Check sheet for the modelled part. Datum: model origin and axes. Units: mm. A direction names the side the tool comes from. Round coordinates to 2 decimals unless told otherwise and drop trailing zeros. Write each loop counter-clockwise with the first axis right and the second up, starting at its lowest first coordinate (ties: lowest second). Pieces come first, ordered by that corner, then holes. Notation, with made-up numbers: M 82,34 L 116,34 A23 ccw 116,53 Z; hole C -29,-17.5 d9. An arc over 180 degrees is marked long. One line per item, written item: value.
from build123d import *

# Parameters (mm, degrees)
BOSS_EXTRUDE1_DEPTH     = 6.35
SKETCH3_R               = 2.286
CUT_EXTRUDE2_DEPTH      = 288.438345563
SKETCH4_R               = 2.286
CUT_EXTRUDE3_DEPTH      = 288.438345563
SKETCH5_W               = 176.1617
SKETCH5_H               = 113.89106
SKETCH5_R               = 2.286
BOSS_EXTRUDE2_DEPTH     = 6.35
FILLET1_R               = 6.35
BOSS_EXTRUDE3_DEPTH     = 6.35
SKETCH8_R               = 4.826
SKETCH8_R_2             = 2.286
BOSS_EXTRUDE4_DEPTH     = 6.35
SKETCH9_R               = 3.8354
CUT_EXTRUDE4_DEPTH      = 3.81
SKETCH10_R              = 1.8034
CUT_EXTRUDE5_DEPTH      = 288.547744905
CUT_EXTRUDE6_DEPTH      = 288.438345563
CUT_EXTRUDE6_DEPTH_BACK = 288.438345563
SKETCH11_R              = 2.286


with BuildPart() as part:
    # Sketch1 → Boss-Extrude1 (new body)
    with BuildSketch(Plane(origin=(0, 0, 0), x_dir=(1, 0, 0), z_dir=(0, 1, 0))):
        Polygon((0, 196.85), (6.35, 203.2), (196.85, 203.2), (203.2, 196.85), (203.2, 6.35), (196.85, 0), (6.35, 0), (0, 6.35), align=None)
    extrude(amount=BOSS_EXTRUDE1_DEPTH)

    # Sketch3 → Cut-Extrude2 (cut, through all)
    with BuildSketch(Plane(origin=(0, 6.35, 0), x_dir=(1, 0, 0), z_dir=(0, 1, 0))):
        with Locations(Location((11.73734, 11.73734, 0), (0, 0, 270))):
            Circle(SKETCH3_R)
        with Locations(Location((191.46266, 11.73734, 0), (0, 0, 270))):
            Circle(SKETCH3_R)
        with Locations(Location((191.46266, 191.46266, 0), (0, 0, 270))):
            Circle(SKETCH3_R)
        with Locations(Location((11.73734, 191.46266, 0), (0, 0, 270))):
            Circle(SKETCH3_R)
    extrude(amount=-CUT_EXTRUDE2_DEPTH, mode=Mode.SUBTRACT)

    # Sketch4 → Cut-Extrude3 (cut, through all)
    with BuildSketch(Plane(origin=(0, 6.35, 0), x_dir=(1, 0, 0), z_dir=(0, 1, 0))):
        with Locations(Location((19.86915, 152.19553, 0), (0, 0, 270))):
            Circle(SKETCH4_R)
        with Locations(Location((183.33085, 152.19553, 0), (0, 0, 270))):
            Circle(SKETCH4_R)
        with Locations(Location((183.33085, 51.00447, 0), (0, 0, 270))):
            Circle(SKETCH4_R)
        with Locations(Location((19.86915, 51.00447, 0), (0, 0, 270))):
            Circle(SKETCH4_R)
        Polygon((16.69415, 140.040273879), (66.688363593, 190.034487472), (136.511636407, 190.034487472), (186.50585, 140.040273879), (186.50585, 63.159726121), (136.511636407, 13.165512528), (66.688363593, 13.165512528), (16.69415, 63.159726121), align=None)
    extrude(amount=-CUT_EXTRUDE3_DEPTH, mode=Mode.SUBTRACT)

    # Sketch5 → Boss-Extrude2 (add)
    with BuildSketch(Plane(origin=(0, 6.35, 0), x_dir=(1, 0, 0), z_dir=(0, 1, 0))):
        with Locations((101.6, 101.6)):
            Rectangle(SKETCH5_W, SKETCH5_H)
        with Locations(Location((183.33085, 51.00447, 0), (0, 0, 270))):
            Circle(SKETCH5_R, mode=Mode.SUBTRACT)
        with Locations(Location((183.33085, 152.19553, 0), (0, 0, 270))):
            Circle(SKETCH5_R, mode=Mode.SUBTRACT)
        with Locations(Location((19.86915, 152.19553, 0), (0, 0, 270))):
            Circle(SKETCH5_R, mode=Mode.SUBTRACT)
        with Locations(Location((19.86915, 51.00447, 0), (0, 0, 270))):
            Circle(SKETCH5_R, mode=Mode.SUBTRACT)
        with BuildLine():
            Line((141.073627551, 145.84553), (62.126372449, 145.84553))
            ThreePointArc((62.126372449, 145.84553), (55.998680779, 141.161031366), (58.911985411, 134.019197653))
            Line((58.911985411, 134.019197653), (98.385612962, 110.849764408))
            ThreePointArc((98.385612962, 110.849764408), (101.6, 109.976096755), (104.814387038, 110.849764408))
            Line((104.814387038, 110.849764408), (144.288014589, 134.019197653))
            ThreePointArc((144.288014589, 134.019197653), (147.201319221, 141.161031366), (141.073627551, 145.84553))
        make_face(mode=Mode.SUBTRACT)
        with BuildLine():
            Line((26.21915, 127.3922384), (26.21915, 75.8077616))
            ThreePointArc((26.21915, 75.8077616), (29.413904977, 70.297141957), (35.783537038, 70.331429253))
            Line((35.783537038, 70.331429253), (79.725622352, 96.123667653))
            ThreePointArc((79.725622352, 96.123667653), (82.861235314, 101.6), (79.725622352, 107.076332347))
            Line((79.725622352, 107.076332347), (35.783537038, 132.868570747))
            ThreePointArc((35.783537038, 132.868570747), (29.413904977, 132.902858043), (26.21915, 127.3922384))
        make_face(mode=Mode.SUBTRACT)
        with BuildLine():
            Line((62.126372449, 57.35447), (141.073627551, 57.35447))
            ThreePointArc((141.073627551, 57.35447), (147.201319221, 62.038968634), (144.288014589, 69.180802347))
            Line((144.288014589, 69.180802347), (104.814387038, 92.350235592))
            ThreePointArc((104.814387038, 92.350235592), (101.6, 93.223903245), (98.385612962, 92.350235592))
            Line((98.385612962, 92.350235592), (58.911985411, 69.180802347))
            ThreePointArc((58.911985411, 69.180802347), (55.998680779, 62.038968634), (62.126372449, 57.35447))
        make_face(mode=Mode.SUBTRACT)
        with BuildLine():
            Line((176.98085, 75.8077616), (176.98085, 127.3922384))
            ThreePointArc((176.98085, 127.3922384), (173.786095023, 132.902858043), (167.416462962, 132.868570747))
            Line((167.416462962, 132.868570747), (123.474377648, 107.076332347))
            ThreePointArc((123.474377648, 107.076332347), (120.338764686, 101.6), (123.474377648, 96.123667653))
            Line((123.474377648, 96.123667653), (167.416462962, 70.331429253))
            ThreePointArc((167.416462962, 70.331429253), (173.786095023, 70.297141957), (176.98085, 75.8077616))
        make_face(mode=Mode.SUBTRACT)
    extrude(amount=-BOSS_EXTRUDE2_DEPTH)

    # Fillet1
    fillet1_edges = [part.edges().sort_by_distance(p)[0] for p in [
        (66.688363593, 3.175, -190.034487472),
        (136.511636407, 3.175, -190.034487472),
        (136.511636407, 3.175, -13.165512528),
        (66.688363593, 3.175, -13.165512528),
        (35.199406121, 3.175, -44.65447),
        (168.000593879, 3.175, -158.54553),
        (35.199406121, 3.175, -158.54553),
        (168.000593879, 3.175, -44.65447),
    ]]
    fillet(fillet1_edges, radius=FILLET1_R)

    # Sketch6 → Boss-Extrude3 (add)
    with BuildSketch(Plane(origin=(0, 6.35, 0), x_dir=(1, 0, 0), z_dir=(0, 1, 0))):
        with BuildLine():
            Line((87.718434183, 13.165512528), (115.481565817, 13.165512528))
            ThreePointArc((115.481565817, 13.165512528), (109.663032532, 15.149272881), (106.268137177, 20.274243151))
            ThreePointArc((106.268137177, 20.274243151), (101.6, 23.876), (96.931862823, 20.274243151))
            ThreePointArc((96.931862823, 20.274243151), (93.536967468, 15.149272881), (87.718434183, 13.165512528))
        make_face()
    extrude(amount=-BOSS_EXTRUDE3_DEPTH)

    # Sketch8 → Boss-Extrude4 (add)
    with BuildSketch(Plane(origin=(0, 0, 0), x_dir=(1, 0, 0), z_dir=(0, 1, 0))):
        with Locations(Location((101.6, 19.05, 0), (0, 0, 270))):
            Circle(SKETCH8_R)
        with Locations(Location((101.6, 19.05, 0), (0, 0, 270))):
            Circle(SKETCH8_R_2, mode=Mode.SUBTRACT)
    extrude(amount=-BOSS_EXTRUDE4_DEPTH)

    # Sketch9 → Cut-Extrude4 (cut)
    with BuildSketch(Plane(origin=(0, 0, 0), x_dir=(1, 0, 0), z_dir=(0, 1, 0))):
        with Locations(Location((81.536660016, 114.02022223, 0), (0, 0, 90))):
            Circle(SKETCH9_R)
        with Locations(Location((121.663339984, 114.02022223, 0), (0, 0, 90))):
            Circle(SKETCH9_R)
        with Locations(Location((121.663339984, 89.17977777, 0), (0, 0, 90))):
            Circle(SKETCH9_R)
        with Locations(Location((81.536660016, 89.17977777, 0), (0, 0, 90))):
            Circle(SKETCH9_R)
    extrude(amount=CUT_EXTRUDE4_DEPTH, mode=Mode.SUBTRACT)

    # Sketch10 → Cut-Extrude5 (cut, through all)
    with BuildSketch(Plane(origin=(0, 3.81, 0), x_dir=(-1, 0, 0), z_dir=(0, -1, 0))):
        with Locations(Location((-81.536660016, 114.02022223, 0), (0, 0, 90))):
            Circle(SKETCH10_R)
        with Locations(Location((-121.663339984, 114.02022223, 0), (0, 0, 90))):
            Circle(SKETCH10_R)
        with Locations(Location((-121.663339984, 89.17977777, 0), (0, 0, 90))):
            Circle(SKETCH10_R)
        with Locations(Location((-81.536660016, 89.17977777, 0), (0, 0, 90))):
            Circle(SKETCH10_R)
    extrude(amount=-CUT_EXTRUDE5_DEPTH, mode=Mode.SUBTRACT)

    # Sketch11 → Cut-Extrude6 (cut, two sides: drawn at the far end of the back side and taken through both)
    with BuildSketch(Plane.XZ.offset(-CUT_EXTRUDE6_DEPTH_BACK)):
        with Locations(Location((31.75, -12.7, 0), (0, 0, 270))):
            Circle(SKETCH11_R)
        with Locations(Location((171.45, -12.7, 0), (0, 0, 270))):
            Circle(SKETCH11_R)
        with Locations(Location((171.45, -190.5, 0), (0, 0, 270))):
            Circle(SKETCH11_R)
        with Locations(Location((31.75, -190.5, 0), (0, 0, 270))):
            Circle(SKETCH11_R)
    extrude(amount=CUT_EXTRUDE6_DEPTH + CUT_EXTRUDE6_DEPTH_BACK, mode=Mode.SUBTRACT)


solid = part.part
Q1. Scan lines: line 1 (X direction, y = 2.75, z = -134); line 2 (X direction, y = 3.5, z = -127.5); line 3 (Z direction, x = 103, y = 5). Record each from-to range of solid material in increasing order. Write a range as [from, to].
Completed:
line 1: [0, 58.94], [144.26, 203.2]
line 2: [0, 26.22], [44.93, 70.02], [133.18, 158.27], [176.98, 203.2]
line 3: [-203.2, -190.03], [-158.55, -145.85], [-110.13, -93.07], [-57.35, -44.65], [-23.67, 0]
Q2. Sectioned sample at A-A on x = 109. Enter the section's corners in (y, z), and give its area (3 significant figures).
Completed:
outline: M 0,-203.2 L 6.35,-203.2 L 6.35,-190.03 L 0,-190.03 Z; M 0,-158.55 L 6.35,-158.55 L 6.35,-145.85 L 0,-145.85 Z; M 0,-113.31 L 6.35,-113.31 L 6.35,-89.89 L 0,-89.89 Z; M 0,-57.35 L 6.35,-57.35 L 6.35,-44.65 L 0,-44.65 Z; M 0,-15.71 L 6.35,-15.71 L 6.35,0 L 0,0 Z
area: 493 mm^2
Q3. Draft check along Z on faces 4 (the flat face through (3.22, 3.13, -3.13)), 5 (the flat face through (203.2, 3, -103)), 6 (the flat face through (26.219, 3, -102)). Enter one of: pulls with the +Z half, pulls with the -Z half, needs draft (parallel to the pull), parting line crosses it, or undercut.
Completed:
face 4: pulls with the +Z half
face 5: needs draft
face 6: undercut
Q4. Sectioned sample at C-C on y = -3. Enter the section's corners in (x, z).
Completed:
outline: C 101.6,-19.05 d9.65; hole C 101.6,-19.05 d4.57
Q5. Sectioned sample at D-D on z = -104.5. Enter the section's corners in (x, y).
Completed:
outline: M 0,0 L 26.22,0 L 26.22,6.35 L 0,6.35 Z; M 82.16,0 L 121.04,0 L 121.04,6.35 L 82.16,6.35 Z; M 176.98,0 L 203.2,0 L 203.2,6.35 L 176.98,6.35 Z
Q6. Access from +Z, -Z, +X, -X, +Y, -Y to the whole of each face (thin tool, end or side, straight path). Record for faces 1 (the flat face through (122, 3.81, -87)), 2 (the cylindrical face through (136.34, 3.13, -13.66)), 3 (the flat face through (103, -6.35, -17)).
Completed:
face 1: -Y
face 2: +Y, -Y
face 3: +Z, -Z, +X, -X, -Y
Q7. Depth check by flat-ended pin: P1, Ø3.5, axis at x = 31.75, z = -190.5, coming from the +Y side; P2, Ø5, axis at x = 170.5, z = -183, coming from the -Y side. Enter the tip coordinate at first touch or a pass-through.
Completed:
P1: through
P2: y = 0
Q8. Sectioned sample at B-B on z = -137. Enter the section's corners in (x, y).
Completed:
outline: M 0,0 L 56.29,0 L 56.29,6.35 L 0,6.35 Z; M 146.91,0 L 203.2,0 L 203.2,6.35 L 146.91,6.35 Z
